```python
from build123d import *

# Parameters (mm, degrees)
SKETCH1_W           = 40
SKETCH1_H           = 40
BOSS_EXTRUDE1_DEPTH = 35.33
SKETCH2_R           = 12.07
CUT_EXTRUDE1_DEPTH  = 42
SKETCH3_W           = 40
SKETCH3_H           = 40
BOSS_EXTRUDE2_DEPTH = 60
CHAMFER1_SIZE       = 30
CHAMFER1_SIZE2      = 17.320508076
CHAMFER2_SIZE       = 3


with BuildPart() as part:
    # Sketch1 → Boss-Extrude1 (new body)
    with BuildSketch(Plane(origin=(0, 0, 0), x_dir=(1, 0, 0), z_dir=(0, 1, 0))):
        Rectangle(SKETCH1_W, SKETCH1_H)
    extrude(amount=BOSS_EXTRUDE1_DEPTH)

    # Sketch2 → Cut-Extrude1 (cut)
    with BuildSketch(Plane(origin=(0, 35.33, 0), x_dir=(1, 0, 0), z_dir=(0, 1, 0))):
        with Locations((-12.07, 0)):
            Circle(SKETCH2_R)
    extrude(amount=-CUT_EXTRUDE1_DEPTH, mode=Mode.SUBTRACT)

    # Sketch3 → Boss-Extrude2 (add)
    with BuildSketch(Plane.XZ):
        Rectangle(SKETCH3_W, SKETCH3_H)
    extrude(amount=BOSS_EXTRUDE2_DEPTH)

    # Chamfer1
    chamfer1_edges = [part.edges().sort_by_distance(p)[0] for p in [
        (20, 35.33, 0),
    ]]
    chamfer1_side = [part.faces().sort_by_distance(p)[0] for p in [
        (20, -12.335, 0),
    ]]
    chamfer(chamfer1_edges, length=CHAMFER1_SIZE, length2=CHAMFER1_SIZE2, reference=chamfer1_side[0])

    # Chamfer2
    chamfer2_edges = [part.edges().sort_by_distance(p)[0] for p in [
        (-20, 35.33, -14.549725266),
        (-20, 35.33, 14.549725266),
        (-8.660254038, 35.33, 20),
        (-8.660254038, 35.33, -20),
    ]]
    chamfer(chamfer2_edges, length=CHAMFER2_SIZE)


solid = part.part
```
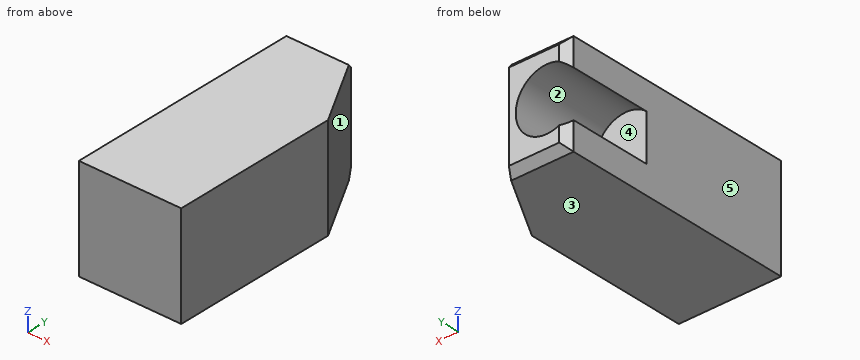
The model under review builds one solid part; all positions refer to its coordinate system, in mm. Face numbers are marked on the shaded views. A direction names the side the tool comes from. Round coordinates to 2 decimals unless told otherwise and drop trailing zeros. Write each loop counter-clockwise with the first axis right and the second up, starting at its lowest first coordinate (ties: lowest second). Pieces come first, ordered by that corner, then holes. Notation, with made-up numbers: (79, -28.5) - (127, -28.5) arc R18 ccw to (127, -9.5) - close; hole circle Ø3 at (80, -18.5). An arc over 180 degrees is marked (long way). One line per question, with ' | ' between items.
Item 1: Add section B-B, the plane x = -12.07. Give the boundary of the cut face in (y, z), then the cut area to 3 significant figures.
Resolved:
outline: (-60, -20) - (32.33, -20) - (35.33, -17) - (35.33, -12.07) - (0, -12.07) - (0, 12.07) - (35.33, 12.07) - (35.33, 17) - (32.33, 20) - (-60, 20) - close | area: 2,950 mm2
Item 2: For the marked faces 1 and 2, list the 3-axis set-ups (+Z, -Z, +X, -X, +Y, -Y) from which the entire face can be reached by the end or side of a thin tool; tool diameter is ignored.
Resolved:
face 1: +Z, -Z, +X, +Y | face 2: +Y
Item 3: Add section A-A, the plane z = 0. Give the boundary of the cut face in (x, y), then the cut area to 3 significant figures.
Resolved:
outline: (-20, -60) - (20, -60) - (20, 5.33) - (2.68, 35.33) - (0, 35.33) - (0, 0) - (-20, 0) - close | area: 2,850 mm2
Item 4: For P1, Ø1, axis at y = 16, z = -12.5, coming from the +X side; P2, Ø16, axis at x = -13, z = -1, coming from the +Y side, all flat-tipped, find the tip position at first contact; note any pin that passes through.
Resolved:
P1: stops at x = 14.13 | P2: stops at y = 0
Item 5: Add section D-D, the plane z = 13.5. Give the boundary of the cut face in (x, y), then the cut area to 3 significant figures.
Resolved:
outline: (-20, -60) - (20, -60) - (20, 5.33) - (2.68, 35.33) - (-17, 35.33) - (-20, 32.33) - close | area: 3,550 mm2
Item 6: The part is to be moulded in two halves that separate along Z. For the marked faces 3, 4 and 5, say which applies: pulls with the +Z half, pulls with the -Z half, needs draft (parallel to the pull), parting line crosses it, or undercut.
Resolved:
face 3: pulls with the -Z half | face 4: undercut | face 5: needs draft
Item 7: To check wall thickness, follow probe 1 along Z at (x, y) = (-12.07, 22); probe 2 along Y at (x, z) = (-3.5, 3); probe 3 along X at (y, z) = (31, -14). State the ranges of each line that lie inside material, in increasing order.
Resolved:
probe 1: z = -20 to -12.07, 12.07 to 20 | probe 2: y = -60 to 0 | probe 3: x = -20 to 5.18
Item 8: Add section C-C, the plane y = 4. Give the boundary of the cut face in (x, z).
Resolved:
outline: (-20, -20) - (20, -20) - (20, 20) - (-20, 20) - (-20, 9.1) arc R12.07 cw (long way) to (-20, -9.1) - close
